Geometry check sheet. Reference: the model listing, model coordinates, mm. A direction names the side the tool comes from. Round coordinates to 2 decimals unless told otherwise and drop trailing zeros. Loops run counter-clockwise (first coordinate to the right, second up) from the corner with the lowest first, then second, coordinate; pieces in that order, holes last.
Autodesk Inventor part; units mm, degrees
ref_plane "YZ Plane" through (0, 0, 0) normal (1, 0, 0) x (0, 1, 0)
ref_plane "XZ Plane" through (0, 0, 0) normal (0, 1, 0) x (-1, 0, 0)
ref_plane "XY Plane" through (0, 0, 0) normal (0, 0, 1) x (1, 0, 0)
sketch "Sketch1" plane through (0, 0, 0) normal (0, 0, 1) x (1, 0, 0)
  line L0 (0, 0) -> (0, 2.413)
  line L1 (0, 2.413) -> (8.382, 2.413)
  line L2 (8.382, 2.413) -> (8.382, 3.175)
  line L3 (8.382, 3.175) -> (9.652, 3.175)
  line L4 (9.652, 3.175) -> (9.652, 3.683)
  line L5 (9.652, 3.683) -> (0.254, 3.683)
  line L6 (0.254, 3.683) -> (0.254, 4.953)
  line L7 (0.254, 4.953) -> (-1.524, 4.953)
  line L8 (-1.524, 4.953) -> (-1.524, 3.683)
  line L9 (0, 0) -> (-1.778, 0)
  line L10 (-1.778, 0) -> (-1.778, 2.413)
  line L11 (-1.778, 2.413) -> (-6.604, 2.413)
  line L12 (-6.604, 2.413) -> (-6.604, 3.175)
  line L13 (-6.604, 3.175) -> (-12.954, 3.175)
  line L14 (-12.954, 3.175) -> (-12.954, 3.81)
  line L15 (-12.954, 3.81) -> (-11.684, 3.81)
  line L16 (-11.684, 3.81) -> (-11.684, 3.556)
  line L17 (-11.684, 3.556) -> (-1.524, 3.683)
  dimension "d0" = 2.413
  dimension "d1" = 8.382
  dimension "d2" = 0.762
  dimension "d3" = 1.27
  dimension "d4" = 0.508
  dimension "d5" = 9.398
  dimension "d6" = 1.27
  dimension "d7" = 1.778
  dimension "d8" = 1.27
  dimension "d9" = 1.778
  dimension "d10" = 2.413
  dimension "d11" = 4.826
  dimension "d12" = 0.762
  dimension "d13" = 6.35
  dimension "d14" = 0.635
  dimension "d15" = 1.27
  dimension "d16" = 0.254
revolve "Revolution1" add sketch "Sketch1" angle 360 about axis through (0, 0, 0) along (-1, 0, 0)
sketch "Sketch2" plane through (-12.954, 0, 0) normal (-1, 0, 0) x (0, 0, 1)
  circle A0 centre (0, 0) radius 3.81
  line L0 (-0.508, 4.1374) -> (0.508, 4.1374)
  line L1 (0.508, 4.1374) -> (0.508, -4.4161)
  line L2 (0.508, -4.4161) -> (-0.508, -4.4161)
  line L3 (-0.508, -4.4161) -> (-0.508, 4.1374)
  dimension "d18" = 1.016
extrude "Extrusion1" cut sketch "Sketch2" against normal blind 5.08 contours L1 A0 L3 | A0 L3 L0 L1 | L1 L2 L3 A0
properties part number "AxleNT"
1) Sectioned sample at A-A, the plane x = -9.5. Record the cut outline in (y, z) (3 decimals).
Report:
outline: (-3.547, -0.508) arc R3.583 ccw to (3.547, -0.508) - (3.134, -0.508) arc R3.175 cw to (-3.134, -0.508) - close; (-3.547, 0.508) - (-3.134, 0.508) arc R3.175 cw to (3.134, 0.508) - (3.547, 0.508) arc R3.583 ccw to start
2) Scan lines: line 1 along Z through (x, y) = (6, 0); line 2 along Y through (x, z) = (9.3, 0) (3 decimals). Record each from-to range of solid material in increasing order.
Report:
line 1: z = -3.68 to -2.41, 2.41 to 3.68
line 2: y = -3.683 to -3.175, 3.175 to 3.683
3) Sectioned sample at C-C, the plane x = -2. Record the cut outline in (y, z), then the cut area to 3 significant figures.
Report:
outline: circle Ø7.35 at (0, 0); hole circle Ø4.83 at (0, 0)
area: 24.2 mm2
4) Mould release check, pull along Y, two halves, no side actions. Record for faces 6 (the face through (-1.778, 0, 0)), 7 (the face through (-12.954, 0, 3.4)), 8 (the face through (-0.65, -0.64, -4.91)): +Y half, -Y half, draft (parallel to the pull), parting line (faces both ways), or undercut.
Report:
face 6: undercut
face 7: draft
face 8: parting line
5) Access from +Z, -Z, +X, -X, +Y, -Y to the whole of each face (thin tool, end or side, straight path). Record for faces 1 (the face through (-6.533, 3.453, 1.087)), 2 (the face through (4.887, 1.699, 3.267)), 3 (the face through (-12.31, -0.08, -3.81)), 4 (the face through (-4.225, -1.915, 1.468)), 5 (the face through (-12.31, 0.08, 3.81)).
Report:
face 1: none
face 2: +X
face 3: -Z, -X
face 4: -X
face 5: +Z, -X
6) Sectioned sample at B-B, the plane x = -4.75. Record the cut outline in (y, z).
Report:
outline: circle Ø7.29 at (0, 0); hole circle Ø4.83 at (0, 0)
7) Gauge pin test, flat ends, axial feed: pin 1 (3 mm diameter, centred on x = -7, y = 2.5, fed in from +Z); pin 2 (4 mm diameter, centred on y = -1, z = 0.5, fed in from +X); pin 3 (1.5 mm diameter, centred on x = -3, z = 0.5, fed in from -Y). Record the tip position at first contact, or that the pin passes through.
Report:
pin 1: stops at z = 3.47
pin 2: stops at x = 8.38
pin 3: stops at y = -3.67
